Autodesk Inventor part; units mm, degrees
ref_plane "YZ Plane" through (0, 0, 0) normal (1, 0, 0) x (0, 1, 0)
ref_plane "XZ Plane" through (0, 0, 0) normal (0, 1, 0) x (-1, 0, 0)
ref_plane "XY Plane" through (0, 0, 0) normal (0, 0, 1) x (1, 0, 0)
sketch "Sketch1" plane through (0, 0, 0) normal (0, 1, 0) x (-1, 0, 0)
  line L0 (0, 0) -> (30.48, 0)
  line L1 (30.48, 0) -> (-30.48, 0)
  line L2 (-30.48, 0) -> (-30.48, -12.192)
  line L3 (-30.48, -12.192) -> (30.48, -12.192)
  line L4 (30.48, -12.192) -> (30.48, 0)
  line L5 (30.48, -12.192) -> (30.48, -11.938)
  line L6 (30.48, -11.938) -> (-30.48, -11.938)
  line L7 (0, 0) -> (0, -7.366)
  circle A0 centre (0, -7.366) radius 2.286
  line L8 (30.48, 0) -> (30.48, 8.89)
  line L9 (30.48, 8.89) -> (-30.48, 8.89)
  line L10 (-30.48, 8.89) -> (-30.48, 0)
  line L11 (30.48, 0) -> (-30.48, 0)
  line L12 (0, 0) -> (0, 4.445)
  circle A1 centre (0, 4.445) radius 2.286
  line L13 (30.48, -12.192) -> (-30.48, -12.192)
  line L14 (-30.48, -12.192) -> (-30.48, -13.2008)
  line L15 (-30.48, -13.2008) -> (30.48, -13.2008)
  line L16 (30.48, -13.2008) -> (30.48, -12.192)
  dimension "d0" = 30.48
  dimension "d1" = 60.96
  dimension "d2" = 12.192
  dimension "d3" = 0.254
  dimension "d4" = 7.366
  dimension "d5" = 4.572
  dimension "d14" = 8.89
  dimension "d15" = 4.572
extrude "Extrusion1" add sketch "Sketch1" along normal blind 9.398 contours L0 L4 L6 L2 L1 | L4 L3 L2 L6
extrude "Extrusion2" add sketch "Sketch1" along normal blind 16.764 contours L16 L15 L14 L3
sketch "Sketch2" plane through (0, 0, 0) normal (0, -1, 0) x (1, 0, 0)
  line L0 (0, 0) -> (0, -7.366)
  circle A0 centre (0, -7.366) radius 3.81
  dimension "d10" = 7.366
  dimension "d11" = 7.62
extrude "Extrusion3" cut sketch "Sketch2" against normal blind 8.89
extrude "Extrusion4" add sketch "Sketch1" along normal blind 9.398 contours L1 L10 L9 L8 L0
sketch "Sketch3" plane through (0, 0, 0) normal (0, -1, 0) x (1, 0, 0)
  line L0 (0, 4.5142) -> (5.0038, 4.5142)
  line L1 (0, 4.5142) -> (-5.0038, 4.5142)
  circle A0 centre (5.0038, 4.5142) radius 1.0109
  circle A1 centre (-5.0038, 4.5142) radius 1.0109
  point P0 (0, 0)
  dimension "d18" = 5.0038
  dimension "d19" = 5.0038
  dimension "d20" = 2.0218
  dimension "d21" = 2.0218
extrude "Extrusion5" cut sketch "Sketch3" against normal blind 4.445
properties part number "VA100CPtoPolarisAdapter"
CAD build for the part. Positions are in the model's coordinates, mm. A direction names the side the tool comes from. Coordinates: 2 decimals unless noted, no trailing zeros. Loops run counter-clockwise (first coordinate to the right, second up) from the corner with the lowest first, then second, coordinate; pieces in that order, holes last. Notation, with made-up numbers: (21, 27) -> (80, 27) arc R16 ccw to (80, 44) -> close; hole circle Ø7 at (30.5, -2). An arc over 180 degrees is marked (long way). One line per item, written item: value.
1. Pull direction Z, two halves, no side cores. Call faces 1 (the face through (-5, 4.445, 5)), 2 (the face through (0, 16.764, -13)), 3 (the face through (2, 8.89, -9)), 4 (the face through (0, 5, 8.89)): pulls with the +Z half, pulls with the -Z half, needs draft (parallel to the pull), parting line crosses it, or undercut.
Answers:
face 1: undercut
face 2: needs draft
face 3: undercut
face 4: pulls with the +Z half
2. Which spindle directions (+Z, -Z, +X, -X, +Y, -Y) get a long thin tool onto all of the face, cutting with end or side? Do faces 5 (the face through (5, 4.445, 5)), 6 (the face through (0, 8, -13.201)), 7 (the face through (0, 13, -12.192)). Say none if no direction does.
Answers:
face 5: -Y
face 6: -Z, +X, -X, +Y, -Y
face 7: +Z, +X, -X, +Y
3. Slice it at C-C on z = -8. Write the cut outline in (x, y), and give its area (3 significant figures).
Answers:
outline: (-30.48, 0) -> (-3.76, 0) -> (-3.76, 8.89) -> (-2.2, 8.89) -> (-2.2, 9.4) -> (-30.48, 9.4) -> close; (2.2, 8.89) -> (3.76, 8.89) -> (3.76, 0) -> (30.48, 0) -> (30.48, 9.4) -> (2.2, 9.4) -> close
area: 504 mm^2
4. Slice it at A-A on x = 0. Write the cut outline in (y, z).
Answers:
outline: (0, -13.2) -> (16.76, -13.2) -> (16.76, -12.19) -> (9.4, -12.19) -> (9.4, -9.65) -> (8.89, -9.65) -> (8.89, -11.18) -> (0, -11.18) -> close; (0, -3.56) -> (8.89, -3.56) -> (8.89, -5.08) -> (9.4, -5.08) -> (9.4, 2.16) -> (0, 2.16) -> close; (0, 6.73) -> (9.4, 6.73) -> (9.4, 8.89) -> (0, 8.89) -> close
5. Flat gauge pins, fed straight in: P1, Ø8, axis at x = -9, y = 14, coming from the +Z side; P2, Ø1, axis at x = 16.5, z = 1.5, coming from the +Y side; P3, Ø2.5, axis at x = -0.5, z = -9, coming from the -Y side. Where does each tip first touch, or does it go through?
Answers:
P1: stops at z = -12.19
P2: stops at y = 9.4
P3: stops at y = 8.89
6. Slice it at B-B on y = 1.75. Write the cut outline in (x, z) (3 decimals), and give its area (3 significant figures).
Answers:
outline: (-30.48, -13.201) -> (30.48, -13.201) -> (30.48, 8.89) -> (-30.48, 8.89) -> close; hole circle Ø2.022 at (-5.004, 4.514); hole circle Ø7.62 at (0, -7.366); hole circle Ø4.572 at (0, 4.445); hole circle Ø2.022 at (5.004, 4.514)
area: 1,280 mm^2
7. Drill centre lines: line 1 (Z direction, x = 0, y = 3.25); line 2 (Z direction, x = 0, y = 9.25); line 3 (X direction, y = 4.25, z = -7.25). Where is each one in solid material? Low to high. Write a range as [from, to].
Answers:
line 1: z = [-13.2, -11.18], [-3.56, 2.16], [6.73, 8.89]
line 2: z = [-13.2, -9.65], [-5.08, 2.16], [6.73, 8.89]
line 3: x = [-30.48, -3.81], [3.81, 30.48]
8. Slice it at D-D on x = 27. Write the cut outline in (y, z), and give its area (3 significant figures).
Answers:
outline: (0, -13.2) -> (16.76, -13.2) -> (16.76, -12.19) -> (9.4, -12.19) -> (9.4, 8.89) -> (0, 8.89) -> close
area: 215 mm^2
